Design review of the part shown in the three views and the two pictorial views. Dimensions are in mm from the part's minimum x, y and z. Give positions to 0.01 mm unless a question says otherwise; leave off trailing zeros. Loops run counter-clockwise (first coordinate to the right, second up) from the corner with the lowest first, then second, coordinate; pieces in that order, holes last.
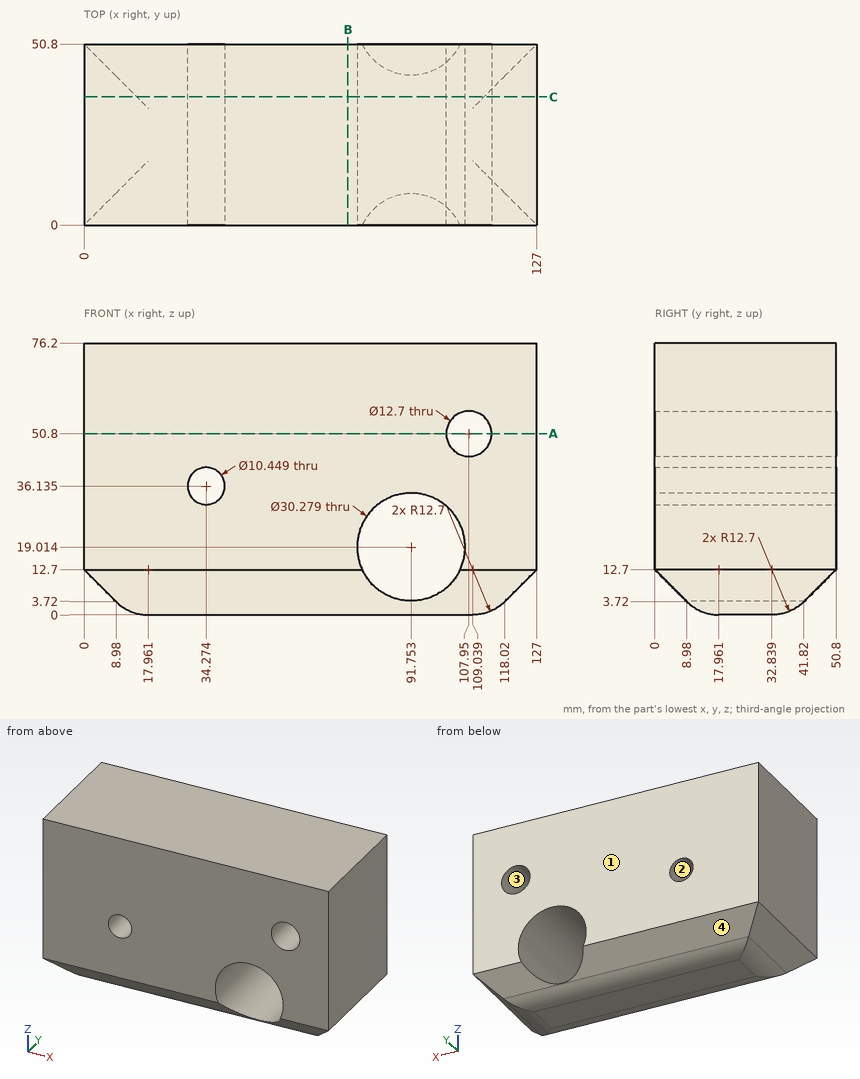
Q1. For pin 1 Ø6 at (x, y) = (111, 8.5) entering from -Z (1 decimal), flat-tipped, find the tip position at first contact; note if it passes through.
Answers:
pin 1: stops at z = 1.8
Q2. For probe 1 along Z at (x, y) = (107.95, 21.5); probe 2 along X at (y, z) = (13, 35) (1 decimal); probe 3 along Z at (x, y) = (67, 33.5), list the stretches that pass through material, from the lowest coordinate up.
Answers:
probe 1: z = 0 to 44.45, 57.15 to 76.2
probe 2: x = 0 to 29.2, 39.4 to 127
probe 3: z = 0.02 to 76.2
Q3. Consider section B-B on x = 74. Give the boundary of the cut face in (y, z).
Answers:
outline: (0, 12.7) - (8.98, 3.72) arc R12.7 ccw to (17.96, 0) - (32.84, 0) arc R12.7 ccw to (41.82, 3.72) - (50.8, 12.7) - (50.8, 76.2) - (0, 76.2) - close
Q4. Consider section A-A on z = 50.8. Give the boundary of the cut face in (x, y).
Answers:
outline: (0, 0) - (101.6, 0) - (101.6, 50.8) - (0, 50.8) - close; (114.3, 0) - (127, 0) - (127, 50.8) - (114.3, 50.8) - close
Q5. Consider section C-C on y = 36. Count the separate pieces of the cut face and the enclosed holes in it, plus the area to 3 significant figures.
Answers:
separate pieces: 1
enclosed holes: 3
area: 8,540 mm2
Q6. Mouldability with a two-part tool opening along Z and no side actions: class the marked faces 1, 2, 3 and 4 as +Z half, -Z half, draft (parallel to the pull), parting line (faces both ways), or undercut.
Answers:
face 1: draft
face 2: undercut
face 3: undercut
face 4: -Z half
